from build123d import *

# Parameters (mm, degrees)
BOSS_EXTRUDE1_DEPTH = 2.54
BOSS_EXTRUDE2_DEPTH = 5.08
SKETCH2_W           = 15.24
SKETCH2_H           = 15.24
SKETCH2_R           = 3.429
BOSS_EXTRUDE3_DEPTH = 5.08
FILLET1_R           = 2.54


with BuildPart() as part:
    # Sketch1 → Boss-Extrude1 (new body)
    with BuildSketch(Plane.XY):
        Polygon((25.4, 0), (25.4, 25.4), (0, 25.4), (0, 0), (-2.54, 0), (-2.54, 27.94), (27.94, 27.94), (27.94, 0), align=None)
        Polygon((0, 25.4), (0, 0), (5.08, 0), (5.08, 20.32), (20.32, 20.32), (20.32, 0), (25.4, 0), (25.4, 25.4), align=None)
    extrude(amount=BOSS_EXTRUDE1_DEPTH)

    # Sketch1_3 → Boss-Extrude2 (add)
    with BuildSketch(Plane.XY):
        Polygon((25.4, 0), (25.4, 25.4), (0, 25.4), (0, 0), (-2.54, 0), (-2.54, 27.94), (27.94, 27.94), (27.94, 0), align=None)
    extrude(amount=-BOSS_EXTRUDE2_DEPTH)

    # Sketch2 → Boss-Extrude3 (add)
    with BuildSketch(Plane.XZ):
        with Locations((35.56, -5.08)):
            Rectangle(SKETCH2_W, SKETCH2_H)
        with Locations(Location((35.56, -5.08, 0), (0, 0, 270))):
            Circle(SKETCH2_R, mode=Mode.SUBTRACT)
    boss_extrude3 = extrude(amount=-BOSS_EXTRUDE3_DEPTH)

    # Mirror1: Boss-Extrude3 across plane
    add(boss_extrude3.mirror(Plane(origin=(12.7, 0, 0), x_dir=(0, 0, 1), z_dir=(1, 0, 0))))

    # Fillet1
    fillet1_edges = [part.edges().sort_by_distance(p)[0] for p in [
        (20.32, 20.32, 1.27),
        (5.08, 20.32, 1.27),
        (5.08, 0, 1.27),
        (-2.54, 27.94, -1.27),
        (27.94, 27.94, -1.27),
        (20.32, 0, 1.27),
        (27.94, 2.54, -12.7),
        (43.18, 2.54, 2.54),
        (43.18, 2.54, -12.7),
        (-2.54, 2.54, -12.7),
        (-17.78, 2.54, -12.7),
        (-17.78, 2.54, 2.54),
    ]]
    fillet(fillet1_edges, radius=FILLET1_R)


solid = part.part
Read the model definition and answer for the solid it produces. Units are mm, in the model's axes. A direction names the side the tool comes from. Coordinates: 2 decimals unless noted, no trailing zeros. Loops run counter-clockwise (first coordinate to the right, second up) from the corner with the lowest first, then second, coordinate; pieces in that order, holes last.
Q1. Consider probe 1 along X at (y, z) = (23.5, -2.5); probe 2 along X at (y, z) = (4.25, -4); probe 3 along Y at (x, z) = (4.5, -5). Determine where each line is inside the solid, lowest interval first.
Q2. Which of the six approach directions +Z, -Z, +X, -X, +Y, -Y give full straight-line access (tool end or side, diameter ignored) to faces 4 (the face through (-2.54, 3, -8)), 5 (the face through (19.596, 19.556, 1.288)), 6 (the face through (27.94, 15, -1))?
Q3. The part is cut by section A-A on x = -10.16. Write down the section's boundary in (y, z), and give its area (3 significant figures).
Q4. The part is cut by section B-B on y = 12.75. Write down the section's boundary in (x, z), and give its area (3 significant figures).
Q5. The mould has two halves that part along X. Classify faces 1 (the face through (-3.264, 2.576, -11.936)), 2 (the face through (32, 5.08, -3)), 3 (the face through (42.416, 2.576, -11.976)): +X half, -X half, draft (parallel to the pull), parting line (faces both ways), or undercut.
Q6. Each of these flat-tipped pins is pushed along its axis until it touches: pin 1 Ø4 at (y, z) = (17.5, -9) entering from +X; pin 2 Ø6 at (y, z) = (16, -1.5) entering from +X; pin 3 Ø5 at (y, z) = (13, -4.5) entering from -X; pin 4 Ø3 at (x, z) = (11, 1.5) entering from -Y. Where does it stop, or does it pass through?
Q7. The part is cut by section D-D on y = 24.5. Write down the section's boundary in (x, z), and give its area (3 significant figures).
Q8. The part is cut by section C-C on z = -3.75. Write down the section's boundary in (x, y), and give its area (3 significant figures).
Results below:
1. probe 1: x = -2.54 to 0, 25.4 to 27.94
1. probe 2: x = -17.78 to -13.41, -6.91 to 0, 25.4 to 32.31, 38.81 to 43.18
1. probe 3: y = 25.4 to 27.94
2. face 4: -Z, +Y, -Y
2. face 5: +Z, -Z, -Y
2. face 6: +Z, -Z, +X, +Y
3. outline: (0, -12.7) - (5.08, -12.7) - (5.08, -8.51) - (0, -8.51) - close; (0, -1.65) - (5.08, -1.65) - (5.08, 2.54) - (0, 2.54) - close
3. area: 42.6 mm2
4. outline: (-2.54, -5.08) - (0, -5.08) - (0, 0) - (5.08, 0) - (5.08, 2.54) - (-2.54, 2.54) - close; (20.32, 0) - (25.4, 0) - (25.4, -5.08) - (27.94, -5.08) - (27.94, 2.54) - (20.32, 2.54) - close
4. area: 64.5 mm2
5. face 1: undercut
5. face 2: draft
5. face 3: +X half
6. pin 1: passes through
6. pin 2: stops at x = 27.94
6. pin 3: stops at x = -2.54
6. pin 4: stops at y = 20.32
7. outline: (-2.54, -5.08) - (0, -5.08) - (0, 0) - (25.4, 0) - (25.4, -5.08) - (27.94, -5.08) - (27.94, 2.54) - (-2.54, 2.54) - close
7. area: 103 mm2
8. outline: (-17.78, 0) - (-13.32, 0) - (-13.32, 5.08) - (-17.78, 5.08) - close; (-7, 0) - (0, 0) - (0, 25.4) - (25.4, 25.4) - (25.4, 0) - (32.4, 0) - (32.4, 5.08) - (27.94, 5.08) - (27.94, 25.4) arc R2.54 ccw to (25.4, 27.94) - (0, 27.94) arc R2.54 ccw to (-2.54, 25.4) - (-2.54, 5.08) - (-7, 5.08) - close; (38.72, 0) - (43.18, 0) - (43.18, 5.08) - (38.72, 5.08) - close
8. area: 294 mm2
